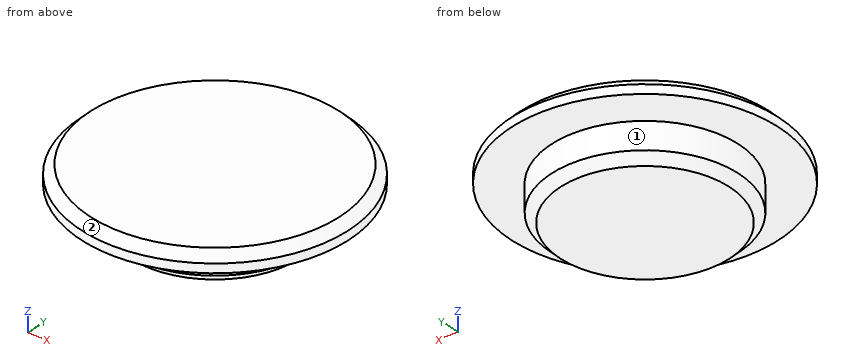
Autodesk Inventor part; units mm, degrees
ref_plane "YZ Plane" through (0, 0, 0) normal (1, 0, 0) x (0, 1, 0)
ref_plane "XZ Plane" through (0, 0, 0) normal (0, 1, 0) x (-1, 0, 0)
ref_plane "XY Plane" through (0, 0, 0) normal (0, 0, 1) x (1, 0, 0)
sketch "Sketch1" plane through (0, 0, 0) normal (0, 0, 1) x (1, 0, 0)
  circle A0 centre (0, 0) radius 10.5
  dimension "d0" = 21
extrude "Extrusion1" add sketch "Sketch1" along normal blind 4
sketch "Sketch2" plane through (0, 0, 4) normal (0, 0, 1) x (1, 0, 0)
  circle A0 centre (0, 0) radius 15
  dimension "d3" = 30
extrude "Extrusion2" add sketch "Sketch2" along normal blind 2
chamfer "Chamfer1" distance 1 angle 45 1 edges at (-15, 0, 6)
chamfer "Chamfer2" distance 1 angle 45 1 edges at (-10.5, 0, 0)
properties part number "Plug21mm_3DPrint"
Part model, mm, in its own coordinate system. Face numbers are marked on the shaded views. A direction names the side the tool comes from. Coordinates: 2 decimals unless noted, no trailing zeros. Loops run counter-clockwise (first coordinate to the right, second up) from the corner with the lowest first, then second, coordinate; pieces in that order, holes last. Notation, with made-up numbers: (-8, -30) - (-2, -30) arc R38 ccw to (-2, 8) - close; hole circle Ø11 at (5, -21.5). An arc over 180 degrees is marked (long way). Write each question's results on one line, items separated by ' | '. Start each with the question number.
Q1. Slice it at D-D on z = 2.7. Give the cut face in (x, y).
Q2. Slice it at A-A on y = 0. Give the cut face in (x, z).
Q3. Which spindle directions (+Z, -Z, +X, -X, +Y, -Y) get a long thin tool onto all of the face, cutting with end or side? Do the marked faces 1 and 2. Say none if no direction does.
Q4. Slice it at C-C on z = 4.4. Give the cut face in (x, y), and give its area (3 significant figures).
Q5. Probe line 1 along Z through (x, y) = (-9, 7.25); line 2 along Y through (x, z) = (0, 4.2); line 3 along X through (y, z) = (1.5, 2.1). List the from-to ranges inside material, lowest first.
Answer:
1) outline: circle Ø21 at (0, 0)
2) outline: (-15, 4) - (-10.5, 4) - (-10.5, 1) - (-9.5, 0) - (9.5, 0) - (10.5, 1) - (10.5, 4) - (15, 4) - (15, 5) - (14, 6) - (-14, 6) - (-15, 5) - close
3) face 1: -Z | face 2: +Z
4) outline: circle Ø30 at (0, 0) | area: 707 mm2
5) line 1: z = 4 to 6 | line 2: y = -15 to 15 | line 3: x = -10.39 to 10.39
